Geometry check sheet. Reference: the model listing, model coordinates, mm. A direction names the side the tool comes from. Coordinates: 2 decimals unless noted, no trailing zeros. Write each loop counter-clockwise with the first axis right and the second up, starting at its lowest first coordinate (ties: lowest second). Pieces come first, ordered by that corner, then holes. Notation, with made-up numbers: M 15,7 L 26,7 A30 ccw 26,35 Z; hole C -23.5,28.25 d10. An arc over 180 degrees is marked long. Answer as a JSON object with one key per item and string values. Group by question number.
```python
from build123d import *

# Parameters (mm, degrees)
SKETCH_1_W          = 10
SKETCH_1_H          = 10
SKETCH_1_W_2        = 8
SKETCH_1_H_2        = 8
EXTRUDE_1_DEPTH     = 51
SKETCH_2_R          = 1.6
CUT_EXTRUDE_1_DEPTH = 53.211109929
SKETCH_3_R          = 1.6
CUT_EXTRUDE_2_DEPTH = 10
SKETCH_4_W          = 10
SKETCH_4_H          = 10
SKETCH_4_W_2        = 8
SKETCH_4_H_2        = 8
EXTRUDE_1_2_DEPTH   = 30
SKETCH_5_R          = 1.6
CUT_EXTRUDE_3_DEPTH = 82.767964387


with BuildPart() as part:
    # ｽｹｯﾁ1 → Extrude 1 (new body)
    with BuildSketch(Plane.XY):
        Rectangle(SKETCH_1_W, SKETCH_1_H)
        Rectangle(SKETCH_1_W_2, SKETCH_1_H_2, mode=Mode.SUBTRACT)
    extrude(amount=EXTRUDE_1_DEPTH)

    # ｽｹｯﾁ2 → ｶｯﾄ - 押し出し1 (cut, through all)
    with BuildSketch(Plane(origin=(5, 0, 0), x_dir=(0, 0, -1), z_dir=(1, 0, 0))):
        with Locations(Location((-36, 0, 0), (0, 0, 90))):
            Circle(SKETCH_2_R)
    extrude(amount=-CUT_EXTRUDE_1_DEPTH, mode=Mode.SUBTRACT)

    # ｽｹｯﾁ3 → ｶｯﾄ - 押し出し2 (cut)
    with BuildSketch(Plane(origin=(0, 5, 0), x_dir=(1, 0, 0), z_dir=(0, 1, 0))):
        with Locations(Location((0, -46, 0), (0, 0, 180))):
            Circle(SKETCH_3_R)
        with Locations(Location((0, -5, 0), (0, 0, 180))):
            Circle(SKETCH_3_R)
    extrude(amount=-CUT_EXTRUDE_2_DEPTH, mode=Mode.SUBTRACT)

    # ｽｹｯﾁ4 → Extrude 1 2 (add)
    with BuildSketch(Plane.XY.offset(51)):
        Rectangle(SKETCH_4_W, SKETCH_4_H)
        Rectangle(SKETCH_4_W_2, SKETCH_4_H_2, mode=Mode.SUBTRACT)
    extrude(amount=EXTRUDE_1_2_DEPTH)

    # ｽｹｯﾁ5 → ｶｯﾄ - 押し出し3 (cut, through all)
    with BuildSketch(Plane(origin=(5, 0, 0), x_dir=(0, 0, -1), z_dir=(1, 0, 0))):
        with Locations(Location((-76, 0, 0), (0, 0, 90))):
            Circle(SKETCH_5_R)
    extrude(amount=-CUT_EXTRUDE_3_DEPTH, mode=Mode.SUBTRACT)


solid = part.part
```
1) Go/stop test with a flat-tipped pin: pin 1 Ø5 at (y, z) = (0, 36) entering from -X. Record where the tip stops, or that it passes through.
2) Section check B-B (x = 0). Record the cut outline in (y, z), then the cut area to 3 significant figures.
3) Material ranges on probe 1 along Z at (x, y) = (0, -4.6); probe 2 along Z at (x, y) = (-4.7, 0); probe 3 along X at (y, z) = (0.75, 47), recorded low to high. Write a range as [from, to].
4) Set-up check for faces 5 (the flat face through (0, 4, 40)), 6 (the cylindrical face through (-0.74, -4.49, 44.58)): record each of +Z, -Z, +X, -X, +Y, -Y from which the full face is reachable in a straight line by a thin tool's end or side.
5) Draft check along Y on faces 1 (the flat face through (0, 5, 40)), 2 (the flat face through (-4, 0, 40)), 3 (the cylindrical face through (0.35, -4.49, 3.44)), 4 (the flat face through (0, -5, 40)). Enter one of: +Y half, -Y half, draft (parallel to the pull), parting line (faces both ways), or undercut.
6) Section check C-C (z = 9.5). Record the cut outline in (x, y).
7) Section check A-A (y = -3). Record the cut outline in (x, z), then the cut area to 3 significant figures.
8) Section check D-D (y = 0). Record the cut outline in (x, z).
Entries:
{
 "1": {"pin 1": "x = -5"},
 "2": {"outline": "M -5,0 L -4,0 L -4,3.4 L -5,3.4 Z; M -5,6.6 L -4,6.6 L -4,44.4 L -5,44.4 Z; M -5,47.6 L -4,47.6 L -4,81 L -5,81 Z; M 4,0 L 5,0 L 5,3.4 L 4,3.4 Z; M 4,6.6 L 5,6.6 L 5,44.4 L 4,44.4 Z; M 4,47.6 L 5,47.6 L 5,81 L 4,81 Z", "area": "149 mm^2"},
 "3": {"probe 1": "[0, 3.4], [6.6, 44.4], [47.6, 81]", "probe 2": "[0, 34.4], [37.6, 74.4], [77.6, 81]", "probe 3": "[-5, -4], [4, 5]"},
 "4": {"face 5": "+Z, -Z", "face 6": "+Y, -Y"},
 "5": {"face 1": "+Y half", "face 2": "undercut", "face 3": "draft", "face 4": "-Y half"},
 "6": {"outline": "M -5,-5 L 5,-5 L 5,5 L -5,5 Z; hole M -4,-4 L 4,-4 L 4,4 L -4,4 Z"},
 "7": {"outline": "M -5,0 L -4,0 L -4,81 L -5,81 Z; M 4,0 L 5,0 L 5,81 L 4,81 Z", "area": "162 mm^2"},
 "8": {"outline": "M -5,0 L -4,0 L -4,34.4 L -5,34.4 Z; M -5,37.6 L -4,37.6 L -4,74.4 L -5,74.4 Z; M -5,77.6 L -4,77.6 L -4,81 L -5,81 Z; M 4,0 L 5,0 L 5,34.4 L 4,34.4 Z; M 4,37.6 L 5,37.6 L 5,74.4 L 4,74.4 Z; M 4,77.6 L 5,77.6 L 5,81 L 4,81 Z"}
}
